```python
from build123d import *

# Parameters (mm, degrees)
SKETCH1_W           = 84
SKETCH1_H           = 80
BOSS_EXTRUDE1_DEPTH = 8
SKETCH2_R           = 12.5
BOSS_EXTRUDE3_DEPTH = 8
FILLET1_R           = 16
SKETCH3_R           = 4
BOSS_EXTRUDE4_DEPTH = 40
SKETCH4_R           = 20
SKETCH4_R_2         = 12.5
BOSS_EXTRUDE5_DEPTH = 8
SKETCH5_R           = 6.5
BOSS_EXTRUDE6_DEPTH = 80
FILLET2_R           = 5
SKETCH6_R           = 16
SKETCH6_R_2         = 5
BOSS_EXTRUDE7_DEPTH = 8


with BuildPart() as part:
    # Sketch1 → Boss-Extrude1 (new body)
    with BuildSketch(Plane(origin=(0, 0, 0), x_dir=(0, 1, 0), z_dir=(0, 0, 1))):
        with Locations((42, 0)):
            Rectangle(SKETCH1_W, SKETCH1_H)
    extrude(amount=BOSS_EXTRUDE1_DEPTH)

    # Sketch2 → Boss-Extrude3 (add)
    with BuildSketch(Plane.YZ.offset(40)):
        with BuildLine():
            Line((0, 0), (0, 40))
            Line((0, 40), (111, 40))
            ThreePointArc((111, 40), (131, 20), (111, 0))
            Line((111, 0), (0, 0))
        make_face()
        with Locations((111, 20)):
            Circle(SKETCH2_R, mode=Mode.SUBTRACT)
    boss_extrude3 = extrude(amount=-BOSS_EXTRUDE3_DEPTH)

    # Mirror1: Boss-Extrude3 across plane
    add(boss_extrude3.mirror(Plane(origin=(0, 0, 0), x_dir=(0, 0, 1), z_dir=(1, 0, 0))))

    # Fillet1
    fillet1_edges = [part.edges().sort_by_distance(p)[0] for p in [
        (-40, 0, 20),
        (40, 0, 20),
    ]]
    fillet(fillet1_edges, radius=FILLET1_R)

    # Sketch3 → Boss-Extrude4 (add)
    with BuildSketch(Plane(origin=(0, 0, 0), x_dir=(0, 1, 0), z_dir=(0, 0, 1))):
        with BuildLine():
            Line((8, 14.202041029), (8, -14.202041029))
            ThreePointArc((8, -14.202041029), (9.433301096, -16.760449625), (12.363636364, -16.874211657))
            ThreePointArc((12.363636364, -16.874211657), (21.656854249, -18.343145751), (23.125788343, -27.636363636))
            ThreePointArc((23.125788343, -27.636363636), (23.239550375, -30.566698904), (25.797958971, -32))
            Line((25.797958971, -32), (84, -32))
            Line((84, -32), (84, -40))
            Line((84, -40), (16, -40))
            ThreePointArc((16, -40), (4.686291501, -35.313708499), (0, -24))
            Line((0, -24), (0, 24))
            ThreePointArc((0, 24), (4.686291501, 35.313708499), (16, 40))
            Line((16, 40), (84, 40))
            Line((84, 40), (84, 32))
            Line((84, 32), (25.797958971, 32))
            ThreePointArc((25.797958971, 32), (23.239550375, 30.566698904), (23.125788343, 27.636363636))
            ThreePointArc((23.125788343, 27.636363636), (21.656854249, 18.343145751), (12.363636364, 16.874211657))
            ThreePointArc((12.363636364, 16.874211657), (9.433301096, 16.760449625), (8, 14.202041029))
        make_face()
        with Locations(Location((16, 24, 0), (0, 0, 90))):
            Circle(SKETCH3_R, mode=Mode.SUBTRACT)
        with Locations(Location((16, -24, 0), (0, 0, 90))):
            Circle(SKETCH3_R, mode=Mode.SUBTRACT)
    extrude(amount=BOSS_EXTRUDE4_DEPTH)

    # Sketch4 → Boss-Extrude5 (add)
    with BuildSketch(Plane.YZ.offset(-32)):
        with Locations(Location((111, 20, 0), (0, 0, 90))):
            Circle(SKETCH4_R)
        with Locations((111, 20)):
            Circle(SKETCH4_R_2, mode=Mode.SUBTRACT)
    boss_extrude5 = extrude(amount=BOSS_EXTRUDE5_DEPTH)

    # Mirror2: Boss-Extrude5 across plane
    add(boss_extrude5.mirror(Plane(origin=(0, 0, 0), x_dir=(0, 0, 1), z_dir=(1, 0, 0))))

    # Sketch5 → Boss-Extrude6 (add)
    with BuildSketch(Plane.YZ.offset(40)):
        with BuildLine():
            Line((52, -15), (52, 0))
            Line((52, 0), (82, 0))
            Line((82, 0), (82, -15))
            ThreePointArc((82, -15), (67, -30), (52, -15))
        make_face()
        with Locations((67, -15)):
            Circle(SKETCH5_R, mode=Mode.SUBTRACT)
    extrude(amount=-BOSS_EXTRUDE6_DEPTH)

    # Fillet2
    # the kernel refuses this fillet: 5 mm, written as the material it adds along each edge
    with BuildSketch(Plane(origin=(40, 82, 0), x_dir=(0, 1, 0), z_dir=(-1, 0, 0))) as fillet2_piece_1_section:
        with BuildLine():
            CenterArc((FILLET2_R, FILLET2_R), FILLET2_R, 180, 90)
            Line((0, FILLET2_R), (0, 0))
            Line((0, 0), (FILLET2_R, 0))
        make_face()
    fillet2_piece_1 = extrude(amount=80, mode=Mode.PRIVATE)
    fillet2_piece_1 = split(fillet2_piece_1, bisect_by=Plane(origin=(32, 84.91705828, -0.211887472), z_dir=(1, 0, 0)), keep=Keep.TOP, mode=Mode.PRIVATE)
    fillet2_piece_1 = split(fillet2_piece_1, bisect_by=Plane(origin=(36, 84, -0.211887472), z_dir=(0, 1, 0)), keep=Keep.TOP, mode=Mode.PRIVATE)
    add(fillet2_piece_1)
    with BuildSketch(Plane(origin=(40, 82, 0), x_dir=(0, 1, 0), z_dir=(-1, 0, 0))) as fillet2_piece_2_section:
        with BuildLine():
            CenterArc((FILLET2_R, FILLET2_R), FILLET2_R, 180, 90)
            Line((0, FILLET2_R), (0, 0))
            Line((0, 0), (FILLET2_R, 0))
        make_face()
    fillet2_piece_2 = extrude(amount=80, mode=Mode.PRIVATE)
    fillet2_piece_2 = split(fillet2_piece_2, bisect_by=Plane(origin=(32, 82.693888299, -1.35777961), z_dir=(1, 0, 0)), keep=Keep.TOP, mode=Mode.PRIVATE)
    fillet2_piece_2 = split(fillet2_piece_2, bisect_by=Plane(origin=(36, 84, -1.35777961), z_dir=(0, -1, 0)), keep=Keep.TOP, mode=Mode.PRIVATE)
    add(fillet2_piece_2)
    with BuildSketch(Plane(origin=(40, 82, 0), x_dir=(0, 1, 0), z_dir=(-1, 0, 0))) as fillet2_piece_3_section:
        with BuildLine():
            CenterArc((FILLET2_R, FILLET2_R), FILLET2_R, 180, 90)
            Line((0, FILLET2_R), (0, 0))
            Line((0, 0), (FILLET2_R, 0))
        make_face()
    fillet2_piece_3 = extrude(amount=80, mode=Mode.PRIVATE)
    fillet2_piece_3 = split(fillet2_piece_3, bisect_by=Plane(origin=(32, 82.693888299, -1.35777961), z_dir=(-1, 0, 0)), keep=Keep.TOP, mode=Mode.PRIVATE)
    fillet2_piece_3 = split(fillet2_piece_3, bisect_by=Plane(origin=(-32, 82.693888299, -1.35777961), z_dir=(1, 0, 0)), keep=Keep.TOP, mode=Mode.PRIVATE)
    fillet2_piece_3 = split(fillet2_piece_3, bisect_by=Plane(origin=(0, 84, -1.35777961), z_dir=(0, -1, 0)), keep=Keep.TOP, mode=Mode.PRIVATE)
    add(fillet2_piece_3)
    with BuildSketch(Plane(origin=(40, 82, 0), x_dir=(0, 1, 0), z_dir=(-1, 0, 0))) as fillet2_piece_4_section:
        with BuildLine():
            CenterArc((FILLET2_R, FILLET2_R), FILLET2_R, 180, 90)
            Line((0, FILLET2_R), (0, 0))
            Line((0, 0), (FILLET2_R, 0))
        make_face()
    fillet2_piece_4 = extrude(amount=80, mode=Mode.PRIVATE)
    fillet2_piece_4 = split(fillet2_piece_4, bisect_by=Plane(origin=(-32, 84.91705828, -0.211887472), z_dir=(-1, 0, 0)), keep=Keep.TOP, mode=Mode.PRIVATE)
    fillet2_piece_4 = split(fillet2_piece_4, bisect_by=Plane(origin=(-36, 84, -0.211887472), z_dir=(0, 1, 0)), keep=Keep.TOP, mode=Mode.PRIVATE)
    add(fillet2_piece_4)
    with BuildSketch(Plane(origin=(40, 82, 0), x_dir=(0, 1, 0), z_dir=(-1, 0, 0))) as fillet2_piece_5_section:
        with BuildLine():
            CenterArc((FILLET2_R, FILLET2_R), FILLET2_R, 180, 90)
            Line((0, FILLET2_R), (0, 0))
            Line((0, 0), (FILLET2_R, 0))
        make_face()
    fillet2_piece_5 = extrude(amount=80, mode=Mode.PRIVATE)
    fillet2_piece_5 = split(fillet2_piece_5, bisect_by=Plane(origin=(-32, 82.693888299, -1.35777961), z_dir=(-1, 0, 0)), keep=Keep.TOP, mode=Mode.PRIVATE)
    fillet2_piece_5 = split(fillet2_piece_5, bisect_by=Plane(origin=(-36, 84, -1.35777961), z_dir=(0, -1, 0)), keep=Keep.TOP, mode=Mode.PRIVATE)
    add(fillet2_piece_5)
    with BuildSketch(Plane(origin=(40, 52, 0), x_dir=(0, -1, 0), z_dir=(-1, 0, 0))) as fillet2_piece_6:
        with BuildLine():
            CenterArc((FILLET2_R, -FILLET2_R), FILLET2_R, 90, 90)
            Line((0, -FILLET2_R), (0, 0))
            Line((0, 0), (FILLET2_R, 0))
        make_face()
    extrude(amount=80)

    # Sketch6 → Boss-Extrude7 (add)
    with BuildSketch(Plane.XZ):
        with Locations(Location((0, 16, 0), (0, 0, 270))):
            Circle(SKETCH6_R)
        with Locations((0, 16)):
            Circle(SKETCH6_R_2, mode=Mode.SUBTRACT)
    extrude(amount=BOSS_EXTRUDE7_DEPTH)


solid = part.part
```
Input: part model. Units: mm. Frame: model coordinates. A direction names the side the tool comes from. Coordinates: 2 decimals unless noted, no trailing zeros. Order: outer loops, then holes, each group sorted by start corner. A loop starts at its lowest first (then second) coordinate and runs counter-clockwise, first axis right, second up. Notation, with made-up numbers: (-38, 84.25) - (-25, 84.25) arc R25 cw to (-25, 114.25) - close; hole circle Ø1 at (70, -18). An arc over 180 degrees is marked (long way). Return JSON: item names as keys, results as strings.
Q1. First-contact query: pin 1 (8 mm diameter, centred on x = 13, z = -10.5, fed in from +Y); pin 2 (4 mm diameter, centred on x = 25.5, y = 16, fed in from +Z); pin 3 (2 mm diameter, centred on x = -10, z = 3, fed in from +Y). Flat tips, straight axial feed; report the tip coordinate or a pass-through.
The answers:
{"pin 1": "stops at y = 82", "pin 2": "stops at z = 8", "pin 3": "stops at y = 84"}
Q2. Draft query along Z for faces 1 (the flat face through (40, 73, 13)), 2 (the cylindrical face through (-1.08, -3.94, 11.12)), 3 (the cylindrical face through (1, 50, -1)), 4 (the flat face through (0, 45, 8)). Return one class per face: +Z half, -Z half, draft (parallel to the pull), parting line (faces both ways), or undercut.
The answers:
{"face 1": "draft", "face 2": "undercut", "face 3": "-Z half", "face 4": "+Z half"}
Q3. Cut plane D-D (z = -6.5). Return loops of the section in (x, y), then the cut area to 3 significant figures.
The answers:
{"outline": "(-40, 52) - (40, 52) - (40, 82) - (-40, 82) - close", "area": "2,400 mm2"}
Q4. Cut plane C-C (y = 103). Return loops of the section in (x, z), then the cut area to 3 significant figures.
The answers:
{"outline": "(-40, 0) - (-32, 0) - (-32, 1.67) - (-24, 1.67) - (-24, 10.4) - (-40, 10.4) - close; (-40, 29.6) - (-24, 29.6) - (-24, 38.33) - (-32, 38.33) - (-32, 40) - (-40, 40) - close; (24, 1.67) - (32, 1.67) - (32, 0) - (40, 0) - (40, 10.4) - (24, 10.4) - close; (24, 29.6) - (40, 29.6) - (40, 40) - (32, 40) - (32, 38.33) - (24, 38.33) - close", "area": "612 mm2"}
Q5. Cut plane B-B (z = 23). State how many separate pieces and enclosed holes the cut face has, then the cut area to 3 significant figures.
The answers:
{"separate pieces": "3", "enclosed holes": "2", "area": "2,950 mm2"}
Q6. Cut plane A-A (y = 67). Return loops of the section in (x, z), then the cut area to 3 significant figures.
The answers:
{"outline": "(-40, -30) - (40, -30) - (40, -21.5) - (-40, -21.5) - close; (-40, -8.5) - (40, -8.5) - (40, 40) - (32, 40) - (32, 8) - (-32, 8) - (-32, 40) - (-40, 40) - close", "area": "2,510 mm2"}
Q7. Access query for faces 5 (the cylindrical face through (30.334, 130.524, 15.664)), 6 (the cylindrical face through (-20, 16, 24)), 7 (the flat face through (-24, 120, 11)). Directions: +Z, -Z, +X, -X, +Y, -Y. A direction counts if a zero-diameter tool reaches every point of the face in a straight line with its end or side. Return the directions, or none.
The answers:
{"face 5": "none", "face 6": "+Z", "face 7": "+Z, -Z, +Y"}
Q8. Ray query, probe 1 along X at (y, z) = (16, 26); probe 2 along Z at (x, y) = (4, 67); probe 3 along Y at (x, z) = (-31, 31.5). Return the intervals inside material, ascending.
The answers:
{"probe 1": "x = -40 to -28, -20 to -16, 16 to 20, 28 to 40", "probe 2": "z = -30 to -21.5, -8.5 to 8", "probe 3": "y = 1.61 to 23.56, 94.64 to 106.1, 115.9 to 127.36"}
